CAD build for the part. Positions are in the model's coordinates, mm. Coordinates: 2 decimals unless noted, no trailing zeros. Order: outer loops, then holes, each group sorted by start corner. A loop starts at its lowest first (then second) coordinate and runs counter-clockwise, first axis right, second up. Notation, with made-up numbers: M 24,12 L 55,12 A15 ccw 55,27 Z; hole C 35.25,54.5 d1. An arc over 180 degrees is marked long. Write item = value, one per line.
Solid Edge part; units mm, degrees
sketch "Sketch1" plane through (0, 0, 0) normal (0, 0, 1) x (1, 0, 0)
  arc A0 (-52, -26) -> (52, -26) centre (0, -26.2795) cw
  line L0 (-52, -26) -> (52, -26)
extrude "Protrusion1" add sketch "Sketch1" against normal blind 32
sketch "Sketch2" plane through (0, -0.1394, 0) normal (0, 0, 1) x (1, 0, 0)
  line L0 (-55.74, -28.2911) -> (55.74, -28.2911)
  line L1 (55.74, -28.2911) -> (55.74, 28.5699)
  line L2 (55.74, 28.5699) -> (-55.74, 28.5699)
  line L3 (-55.74, 28.5699) -> (-55.74, -28.2911)
extrude "Recorte_Extrudado_2" cut sketch "Sketch2" against normal blind 16.3
sketch "Sketch3" plane through (0, -0.1394, -16.3) normal (0, 0, 1) x (1, 0, 0)
  arc A0 (-52, -25.8606) -> (52, -25.8606) centre (0, -26.1401) cw
  line L0 (-52, -25.8606) -> (52, -25.8606)
extrude "Protrusão_Extrudada_6" add sketch "Sketch3" along normal blind 16.3
(1) Pin check, flat tips, straight feed: pin 1 Ø4 at (x, z) = (18, -4.5) entering from +Y; pin 2 Ø5 at (y, z) = (-7.5, -25) entering from -X; pin 3 Ø5 at (y, z) = (16, -25.5) entering from -X. Stop position of each tip, or through.
Evaluation:
pin_1 = 23.2
pin_2 = -49.39
pin_3 = -33.49
(2) Slice it at B-B, the plane x = -9.5. Write the cut outline in (y, z), then the cut area to 3 significant figures.
Evaluation:
outline = M -26,-32 L 24.85,-32 L 24.85,0 L -26,0 Z
area = 1,630 mm²
(3) Wall check: line 1 (Y direction, x = 27.5, z = -21); line 2 (Y direction, x = -30.5, z = -17.5); line 3 (X direction, y = 7, z = -6.5). Give the ranges that are in metal, low to high. Write a range as from..to.
Evaluation:
line_1 = -26..17.85
line_2 = -26..15.84
line_3 = -39.96..39.96
(4) Slice it at C-C, the plane y = -17. Write the cut outline in (x, z), then the cut area to 3 significant figures.
Evaluation:
outline = M -51.17,-32 L 51.17,-32 L 51.17,0 L -51.17,0 Z
area = 3,270 mm²
